```python
from build123d import *

# Parameters (mm, degrees)
SKETCH1_W           = 22.5
SKETCH1_H           = 51
BOSS_EXTRUDE1_DEPTH = 58
CUT_EXTRUDE1_REACH  = 121.301
LPATTERN1_COUNT     = 4
LPATTERN1_PITCH     = 7
LPATTERN1_COL_COUNT = 4
LPATTERN1_COL_PITCH = 7
FILLET1_R           = 0.5
CUT_EXTRUDE2_REACH  = 69.235
SKETCH3_R           = 1


with BuildPart() as part:
    # Sketch1 → Boss-Extrude1 (new, symmetric)
    with BuildSketch(Plane(origin=(0, 0, 0), x_dir=(0, 0, -1), z_dir=(1, 0, 0))):
        Rectangle(SKETCH1_W, SKETCH1_H)
    extrude(amount=BOSS_EXTRUDE1_DEPTH, both=True)

    # Sketch2 → Cut-Extrude1 (cut, up to next)
    with BuildSketch(Plane.ZY.offset(58), mode=Mode.PRIVATE) as cut_extrude1_sk1:
        with BuildLine():
            Line((-4.75, 2.5), (11.25, 2.5))
            Line((11.25, 2.5), (11.25, -2.5))
            Line((11.25, -2.5), (-4.75, -2.5))
            ThreePointArc((-4.75, -2.5), (-7.25, 0), (-4.75, 2.5))
        make_face()
    cut_extrude1_tool1 = extrude(cut_extrude1_sk1.sketch, amount=-CUT_EXTRUDE1_REACH, mode=Mode.PRIVATE) & part.part
    cut_extrude1 = cut_extrude1_tool1.solids().sort_by_distance((-58, 0, 2.259586))[0]
    add(cut_extrude1, mode=Mode.SUBTRACT)

    # LPattern1: Cut-Extrude1 ×4
    with Locations(*[(0, -i * LPATTERN1_PITCH, 0) for i in range(1, LPATTERN1_COUNT)]):
        add(cut_extrude1, mode=Mode.SUBTRACT)

    # LPattern1 col: Cut-Extrude1 ×4
    with Locations(*[(0, i * LPATTERN1_COL_PITCH, 0) for i in range(1, LPATTERN1_COL_COUNT)]):
        add(cut_extrude1, mode=Mode.SUBTRACT)

    # Fillet1
    fillet1_edges = [part.edges().sort_by_distance(p)[0] for p in [
        (0, 2.5, 11.25),
        (0, -2.5, 11.25),
        (0, 9.5, 11.25),
        (0, 4.5, 11.25),
        (0, -18.5, 11.25),
        (0, -23.5, 11.25),
        (0, -4.5, 11.25),
        (0, -9.5, 11.25),
        (0, 23.5, 11.25),
        (0, 18.5, 11.25),
        (0, -25.5, 11.25),
        (0, 25.5, 11.25),
        (0, 16.5, 11.25),
        (0, 11.5, 11.25),
        (0, -11.5, 11.25),
        (0, -16.5, 11.25),
    ]]
    fillet(fillet1_edges, radius=FILLET1_R)

    # Sketch3 → Cut-Extrude2 (cut, up to next)
    with BuildSketch(Plane(origin=(0, 0, -11.25), x_dir=(-1, 0, 0), z_dir=(0, 0, -1)), mode=Mode.PRIVATE) as cut_extrude2_sk1:
        with Locations(Location((-54, 21.5, 0), (0, 0, 90))):
            Circle(SKETCH3_R)
    cut_extrude2_tool1 = extrude(cut_extrude2_sk1.sketch, amount=-CUT_EXTRUDE2_REACH, mode=Mode.PRIVATE) & part.part
    # Sketch3 → Cut-Extrude2 (cut, up to next)
    with BuildSketch(Plane(origin=(0, 0, -11.25), x_dir=(-1, 0, 0), z_dir=(0, 0, -1)), mode=Mode.PRIVATE) as cut_extrude2_sk2:
        with Locations(Location((-54, -21.5, 0), (0, 0, 90))):
            Circle(SKETCH3_R)
    cut_extrude2_tool2 = extrude(cut_extrude2_sk2.sketch, amount=-CUT_EXTRUDE2_REACH, mode=Mode.PRIVATE) & part.part
    # Sketch3 → Cut-Extrude2 (cut, up to next)
    with BuildSketch(Plane(origin=(0, 0, -11.25), x_dir=(-1, 0, 0), z_dir=(0, 0, -1)), mode=Mode.PRIVATE) as cut_extrude2_sk3:
        with Locations(Location((54, -21.5, 0), (0, 0, 90))):
            Circle(SKETCH3_R)
    cut_extrude2_tool3 = extrude(cut_extrude2_sk3.sketch, amount=-CUT_EXTRUDE2_REACH, mode=Mode.PRIVATE) & part.part
    # Sketch3 → Cut-Extrude2 (cut, up to next)
    with BuildSketch(Plane(origin=(0, 0, -11.25), x_dir=(-1, 0, 0), z_dir=(0, 0, -1)), mode=Mode.PRIVATE) as cut_extrude2_sk4:
        with Locations(Location((54, 21.5, 0), (0, 0, 90))):
            Circle(SKETCH3_R)
    cut_extrude2_tool4 = extrude(cut_extrude2_sk4.sketch, amount=-CUT_EXTRUDE2_REACH, mode=Mode.PRIVATE) & part.part
    add(cut_extrude2_tool1.solids().sort_by_distance((54, 21.5, -11.25))[0], mode=Mode.SUBTRACT)
    add(cut_extrude2_tool2.solids().sort_by_distance((54, -21.5, -11.25))[0], mode=Mode.SUBTRACT)
    add(cut_extrude2_tool3.solids().sort_by_distance((-54, -21.5, -11.25))[0], mode=Mode.SUBTRACT)
    add(cut_extrude2_tool4.solids().sort_by_distance((-54, 21.5, -11.25))[0], mode=Mode.SUBTRACT)


solid = part.part
```
Here's how the part is built. I have some questions about the finished solid (model axes, mm). A direction names the side the tool comes from. Coordinates: 2 decimals unless noted, no trailing zeros. Order: outer loops, then holes, each group sorted by start corner. A loop starts at its lowest first (then second) coordinate and runs counter-clockwise, first axis right, second up.
1) Which directions (+Z, -Z, +X, -X, +Y, -Y) give clear straight access to the entire face, cutting with the end or side of a thin tool? Please do faces 4 (the face through (1, 0, -11.25)), 5 (the face through (-1, -4.5, 3)).
2) Imagine slicing it at B-B on y = 14. List the corners of the cut face in (x, z) for me, and give its area (3 significant figures).
3) I need wall thicknesses on line 1 (Y direction, x = -54, z = -8.5); line 2 (X direction, y = 21.5, z = -8.1); line 3 (Z direction, x = -10.5, y = -15.5). Which ranges of each line are inside material? Lowest first, please.
4) Imagine slicing it at C-C on y = -1. List the corners of the cut face in (x, z) for me, and give its area (3 significant figures).
5) We'd pull the mould along X, two halves only. Please class faces 1 (the face through (-1, 2.5, 3)), 2 (the face through (58, -5, -7)), 3 (the face through (-54, -22.5, -9)): +X half, -X half, draft (parallel to the pull), parting line (faces both ways), or undercut.
6) Imagine slicing it at A-A on z = 2.25. State how many separate pieces and enclosed holes the cut face has, and give its area (3 significant figures).
7) Will these pins go through, and if not, where does the flat tip stop? pin 1 (5 mm diameter, centred on x = 25, y = -9, fed in from +Z); pin 2 (2.5 mm diameter, centred on x = 54, y = -21.5, fed in from +Z); pin 3 (1.2 mm diameter, centred on x = -54, y = -21.5, fed in from -Z); pin 4 (1 mm diameter, centred on x = -44, y = -1.5, fed in from +Z).
Response values:
1. face 4: -Z, +X, -X, +Y, -Y
1. face 5: +Z, +X, -X
2. outline: (-58, -11.25) - (58, -11.25) - (58, -7.25) - (-58, -7.25) - close
2. area: 464 mm2
3. line 1: y = -25.5 to -22.5, -20.5 to 20.5, 22.5 to 25.5
3. line 2: x = -58 to -55, -53 to 53, 55 to 58
3. line 3: z = -11.25 to -6.75
4. outline: (-58, -11.25) - (58, -11.25) - (58, -7.04) - (-58, -7.04) - close
4. area: 488 mm2
5. face 1: draft
5. face 2: +X half
5. face 3: undercut
6. separate pieces: 8
6. enclosed holes: 0
6. area: 1,860 mm2
7. pin 1: stops at z = 11.25
7. pin 2: stops at z = -6.54
7. pin 3: passes through
7. pin 4: stops at z = -6.25
